Source: CAD feature listing. Evaluate the final solid. Frame: model axes, mm. A direction names the side the tool comes from. Give positions to 0.01 mm unless a question says otherwise; leave off trailing zeros. Loops run counter-clockwise (first coordinate to the right, second up) from the corner with the lowest first, then second, coordinate; pieces in that order, holes last.
from build123d import *
from build123d.topology import SkipClean

# Parameters (mm, degrees)
BASPROSKE_W             = 10
BASPROSKE_H             = 22
TOOTHCUT_DEPTH          = 33.680269277
TEETHCUTS_COUNT         = 20
TEETHCUTS_ANGLE         = 342
BORSKE_R                = 2
BORE_DEPTH              = 50.0000508
SKETCH3_W               = 21.477286505
SKETCH3_H               = 49.38738346
SKETCH3_W_2             = 5.914035414
SKETCH3_H_2             = 19.713451381
CUT_EXTRUDE1_DEPTH      = 10
SKETCH4_R               = 17.499
SKETCH4_R_2             = 2
BOSS_EXTRUDE2_DEPTH     = 10
BOSS_EXTRUDE3_DEPTH     = 10
CUT_EXTRUDE3_DEPTH      = 56.733338326
CUT_EXTRUDE3_DEPTH_BACK = 56.733338326
SKETCH7_W               = 2
SKETCH7_H               = 71.806333941
SKETCH6_W               = 4
SKETCH6_H               = 4
CUT_EXTRUDE5_DEPTH      = 58.293800183


with BuildPart() as part:
    # BasProSke → Base-Revolve (revolve)
    with BuildSketch(Plane(origin=(0, 0, 0), x_dir=(1, 0, 0), z_dir=(0, 1, 0)), mode=Mode.PRIVATE) as base_revolve_sk:
        with Locations((5, 11)):
            Rectangle(BASPROSKE_W, BASPROSKE_H)
    revolve(base_revolve_sk.sketch.rotate(Axis((-10, 0, 0), (1, 0, 0)), 180), axis=Axis((-10, 0, 0), (1, 0, 0)))

    # TooCutSke → ToothCut (cut, through all)
    with BuildSketch(Plane(origin=(0, 0, 0), x_dir=(0, 0, -1), z_dir=(1, 0, 0))):
        with BuildLine():
            ThreePointArc((0.986171591, 17.471189616), (0, 17.499), (-0.986171591, 17.471189616))
            ThreePointArc((-0.986171591, 17.471189616), (-1.626916196, 19.798789858), (-2.932850173, 21.829260982))
            ThreePointArc((-2.932850173, 21.829260982), (0, 22.0254), (2.932850173, 21.829260982))
            ThreePointArc((2.932850173, 21.829260982), (1.626916196, 19.798789858), (0.986171591, 17.471189616))
        make_face()
    toothcut = extrude(amount=TOOTHCUT_DEPTH, mode=Mode.SUBTRACT)

    # TeethCuts: ToothCut ×20 about axis
    teethcuts_axis = Axis((-10, 0, 0), (1, 0, 0))
    for i in range(1, TEETHCUTS_COUNT):
        add(toothcut.rotate(teethcuts_axis, i * TEETHCUTS_ANGLE / (TEETHCUTS_COUNT - 1)), mode=Mode.SUBTRACT)

    # BorSke → Bore (cut, symmetric)
    with BuildSketch(Plane(origin=(0, 0, 0), x_dir=(0, 0, -1), z_dir=(1, 0, 0))):
        with Locations(Location((0, 0, 0), (0, 0, 180))):
            Circle(BORSKE_R)
    extrude(amount=BORE_DEPTH, both=True, mode=Mode.SUBTRACT)

    # Sketch3 → Cut-Extrude1 (cut)
    with BuildSketch(Plane.ZY):
        with Locations((-15.842569701, 2.389280872)):
            Rectangle(SKETCH3_W, SKETCH3_H)
        Polygon((-0.493085796, 27.082972602), (-5.103926448, 27.082972602), (-5.103926448, 10.689681454), (-0.493085796, 10.689681454), (-0.493085796, 17.471189616), (-0.986171591, 17.471189616), (-0.986171591, 17.499), (-0.493085796, 17.499), align=None)
        with Locations((-2.146908741, -12.447685168)):
            Rectangle(SKETCH3_W_2, SKETCH3_H_2)
    extrude(amount=-CUT_EXTRUDE1_DEPTH, mode=Mode.SUBTRACT)

    # Sketch4 → Boss-Extrude2 (add)
    with SkipClean():  # the faces are left unmerged after this step: merging them gives an invalid solid
        with BuildSketch(Plane.ZY):
            Circle(SKETCH4_R)
            Circle(SKETCH4_R_2, mode=Mode.SUBTRACT)
        extrude(amount=-BOSS_EXTRUDE2_DEPTH)

    # Sketch5 → Boss-Extrude3 (add)
    with BuildSketch(Plane.ZY):
        with BuildLine():
            ThreePointArc((4.460989585, 16.920832513), (4.73110018, 16.847305188), (5, 16.76946633))
            Line((5, 16.76946633), (5, 50))
            Line((5, 50), (-5, 50))
            Line((-5, 50), (-5, 16.76946633))
            ThreePointArc((-5, 16.76946633), (-2.037353312, 17.37999403), (0.986171591, 17.471189616))
            ThreePointArc((0.986171591, 17.471189616), (1.620704589, 19.784848102), (2.912696354, 21.806333941))
            ThreePointArc((2.912696354, 21.806333941), (3.441558231, 21.729143493), (3.968388926, 21.639128664))
            ThreePointArc((3.968388926, 21.639128664), (4.572472634, 19.317333972), (4.460989585, 16.920832513))
        make_face()
        with BuildLine():
            ThreePointArc((-2, 0), (0, 2), (2, 0))
            Line((2, 0), (5, 0))
            Line((5, 0), (5, 16.76946633))
            ThreePointArc((5, 16.76946633), (4.73110018, 16.847305188), (4.460989585, 16.920832513))
            ThreePointArc((4.460989585, 16.920832513), (4.572472634, 19.317333972), (3.968388926, 21.639128664))
            ThreePointArc((3.968388926, 21.639128664), (3.441558231, 21.729143493), (2.912696354, 21.806333941))
            ThreePointArc((2.912696354, 21.806333941), (1.620704589, 19.784848102), (0.986171591, 17.471189616))
            ThreePointArc((0.986171591, 17.471189616), (-2.037353312, 17.37999403), (-5, 16.76946633))
            Line((-5, 16.76946633), (-5, 0))
            Line((-5, 0), (-2, 0))
        make_face()
    extrude(amount=-BOSS_EXTRUDE3_DEPTH)

    # Sketch7 → Cut-Extrude3 (cut, two sides: drawn at the far end of the back side and taken through both)
    with BuildSketch(Plane.XY.offset(5).offset(-CUT_EXTRUDE3_DEPTH_BACK)):
        with Locations((9, 14.096833029)):
            Rectangle(SKETCH7_W, SKETCH7_H)
    extrude(amount=CUT_EXTRUDE3_DEPTH + CUT_EXTRUDE3_DEPTH_BACK, mode=Mode.SUBTRACT)

    # Sketch6 → Cut-Extrude5 (cut, through all)
    with BuildSketch(Plane(origin=(0, 0, -5), x_dir=(-1, 0, 0), z_dir=(0, 0, -1))):
        with Locations((-4, 44)):
            Rectangle(SKETCH6_W, SKETCH6_H)
        with Locations((-4, 32)):
            Rectangle(SKETCH6_W, SKETCH6_H)
    extrude(amount=-CUT_EXTRUDE5_DEPTH, mode=Mode.SUBTRACT)


solid = part.part
1) Cut plane B-B (y = 0). Return loops of the section in (x, z), and give its area (3 significant figures).
Checks:
outline: (0, -17.5) - (8, -17.5) - (8, -2) - (0, -2) - close; (0, 2) - (8, 2) - (8, 17.5) - (0, 17.5) - close
area: 248 mm2
2) Cut plane C-C (y = 31.5). Return loops of the section in (x, z), and give its area (3 significant figures).
Checks:
outline: (0, -5) - (2, -5) - (2, 5) - (0, 5) - close; (6, -5) - (8, -5) - (8, 5) - (6, 5) - close
area: 40.0 mm2
3) Reachability of faces 4 (the cylindrical face through (3.944, 16.992, 10.325)), 5 (the cylindrical face through (3.94, 18.29, 7.63)), 6 (the flat face through (2, 44, 0)), 7 (the cylindrical face through (3.944, 7.678, 18.341)), 8 (the cylindrical face through (3.94, -15.07, 12.97)) from +Z, -Z, +X, -X, +Y, -Y: full face, straight path, thin tool, end or side. Return the list, or none.
Checks:
face 4: +X, -X
face 5: +X, -X, +Y
face 6: +Z, -Z
face 7: +Z, +X, -X
face 8: +X, -X, -Y
4) Ray query, probe 1 along Y at (x, z) = (5, 0); probe 2 along Y at (x, z) = (3.5, -4); probe 3 along Y at (x, z) = (6.25, 0). Return the intervals inside material, ascending.
Checks:
probe 1: y = -17.5 to -2, 2 to 30, 34 to 42, 46 to 50
probe 2: y = -17.04 to 30, 34 to 42, 46 to 50
probe 3: y = -17.5 to -2, 2 to 50
5) Pull-direction query (Z, two-part tool) for faces 1 (the cylindrical face through (3.944, 1.634, 19.816)), 2 (the flat face through (4, 42, 0)), 3 (the cylindrical face through (3.94, -4.57, 19.35)); classes: released by +Z, released by -Z, zero draft, split by the parting line, or undercut.
Checks:
face 1: released by +Z
face 2: zero draft
face 3: undercut
6) Cut plane D-D (z = -6.5). Return loops of the section in (x, y), and give its area (3 significant figures).
Checks:
outline: (0, -16.25) - (8, -16.25) - (8, 16.25) - (0, 16.25) - close
area: 260 mm2
7) Cut plane A-A (z = 0). Return loops of the section in (x, y), and give its area (3 significant figures).
Checks:
outline: (0, -17.5) - (8, -17.5) - (8, -2) - (0, -2) - close; (0, 2) - (8, 2) - (8, 50) - (0, 50) - close; hole (2, 30) - (6, 30) - (6, 34) - (2, 34) - close; hole (2, 42) - (6, 42) - (6, 46) - (2, 46) - close
area: 476 mm2
8) Contact query for flat-ended pins moving along their axis: P1, Ø2, axis at x = 7, y = 28, coming from the +Z side; P2, Ø2, axis at x = 5, y = 6.5, coming from the -Z side; P3, Ø2, axis at x = 4.5, z = -1.5, coming from the -Y side. Output: stop coordinate, or through.
Checks:
P1: stops at z = 5
P2: stops at z = -16.61
P3: stops at y = -17.49
